Autodesk Inventor part; units mm, degrees
ref_plane "Start Plane" through (0, 0, 0) normal (0, 0, 1) x (1, 0, 0)
ref_plane "End Plane" through (0, 0, 406.9182) normal (0, 0, 1) x (1, 0, 0)
ref_plane "YZ Plane" through (0, 0, 0) normal (1, 0, 0) x (0, 1, 0)
ref_plane "Start Plane" through (0, 0, 0) normal (0, 0, 1) x (1, 0, 0)
ref_plane "End Plane" through (0, 0, 406.9182) normal (0, 0, 1) x (1, 0, 0)
sketch "Sketch" plane through (0, 0, 0) normal (0, 0, 1) x (1, 0, 0)
  line L0 (-9.525, -8.0315) -> (-9.525, 8.0315)
  line L1 (-8.0315, 9.525) -> (8.0315, 9.525)
  line L2 (9.525, 8.0315) -> (9.525, -8.0315)
  line L3 (8.0315, -9.525) -> (-8.0315, -9.525)
  arc A0 (-9.525, -8.0315) -> (-8.0315, -9.525) centre (-8.0315, -8.0315) ccw
  arc A1 (-8.0315, 9.525) -> (-9.525, 8.0315) centre (-8.0315, 8.0315) ccw
  arc A2 (9.525, 8.0315) -> (8.0315, 9.525) centre (8.0315, 8.0315) ccw
  arc A3 (8.0315, -9.525) -> (9.525, -8.0315) centre (8.0315, -8.0315) ccw
  arc A4 (-8.0315, 8.2804) -> (-8.2804, 8.0315) centre (-8.0315, 8.0315) ccw
  line L4 (-8.0315, 8.2804) -> (8.0315, 8.2804)
  arc A5 (8.2804, 8.0315) -> (8.0315, 8.2804) centre (8.0315, 8.0315) ccw
  line L5 (8.2804, 8.0315) -> (8.2804, -8.0315)
  arc A6 (8.0315, -8.2804) -> (8.2804, -8.0315) centre (8.0315, -8.0315) ccw
  line L6 (8.0315, -8.2804) -> (-8.0315, -8.2804)
  arc A7 (-8.2804, -8.0315) -> (-8.0315, -8.2804) centre (-8.0315, -8.0315) ccw
  line L7 (-8.2804, -8.0315) -> (-8.2804, 8.0315)
  line L8 (0, 13.768) -> (0, -13.768) construction
  line L9 (-13.8012, 0) -> (13.9669, 0) construction
  dimension "d10" = 19.05
  dimension "d11" = 19.05
  dimension "d12" = 1.2446
  dimension "d15" = 9.525
  dimension "d16" = 9.525
  dimension "d17" = 1.4935
extrude "Body" add sketch "Sketch" along normal up to surface (406.9182 mm away) from surface at 0
sketch "Sketch3" plane through (0, 0, 0) normal (0, 0, 1) x (1, 0, 0)
  line L0 (0, 0) -> (10, 0)
ref_plane "Work Plane3" through (0, 0, 0) normal (0, -1, 0) x (1, 0, 0)
sketch "Sketch5" plane through (9.525, -8.0315, 406.9182) normal (1, 0, 0) x (0, 0, -1)
  circle A0 centre (326.3769, 8.0315) radius 4.7702
  line L0 (0, 16.063) -> (0, 0)
  line L1 (406.9182, 0) -> (0, 0)
  line L2 (406.9182, 16.063) -> (406.9182, 0)
  line L3 (406.9182, 16.063) -> (0, 16.063)
  line L4 (406.9182, 16.063) -> (406.9182, 0)
  point P0 (406.9182, 8.0315)
  point P1 (406.9182, 8.0315)
extrude "Extrusion2" cut sketch "Sketch5" against normal through all contours A0
sketch "Sketch4" plane through (0, 0, 0) normal (0, -1, 0) x (1, 0, 0)
  line L0 (-2, 0) -> (12, 0)
  line L1 (-2, 406.9182) -> (12, 406.9182)
  dimension "d19" = 406.9182
equation "\"d10\" = G_H"
equation "\"d11\" = G_W"
equation "\"d12\" = G_T"
equation "\"d15\" = 0.5 * d10"
equation "\"d16\" = 0.5 * d11"
equation "\"d17\" = G_IR"
equation "\"d3\" = G_L"
equation "\"G_W\" = 19.05"
equation "\"G_H\" = 19.05"
equation "\"G_T\" = 1.2446"
equation "\"G_IR\" = 1.2 * G_T"
equation "\"G_L\" = d19"
equation "\"G_OFFSET_START\" = 0"
equation "\"G_OFFSET_END\" = 0"
equation "\"d14\" = G_OFFSET_END + B_L"
equation "\"B_L\" = 406.91824"
properties part number "ASTM A513 - 3/4 x 3/4 x 49/1000 - 16.02" material "Steel, Mild"
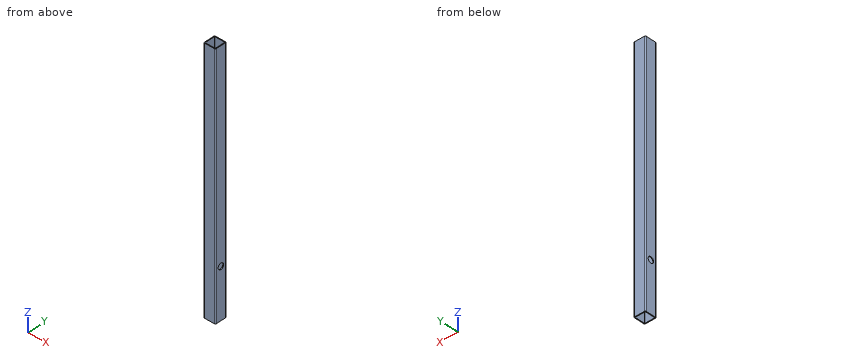
Here's how the part is built. I have some questions about the finished solid (model axes, mm). Round coordinates to 2 decimals unless told otherwise and drop trailing zeros. Loops run counter-clockwise (first coordinate to the right, second up) from the corner with the lowest first, then second, coordinate; pieces in that order, holes last.
1. If I drill on line 1 along X through (y, z) = (-7.5, 262.5) (3 decimals); line 2 along Z through (x, y) = (-8.5, -2), over which ranges is the centre line in solid material (lowest first)?
Answer list:
line 1: x = -9.525 to -8.28, 8.28 to 9.525
line 2: z = 0 to 76.21, 84.87 to 406.92
2. If we section it at A-A on x = -1.25: Write out the boundary of the cut face in (y, z) (3 decimals).
Answer list:
outline: (-9.525, 0) - (-8.28, 0) - (-8.28, 406.918) - (-9.525, 406.918) - close; (8.28, 0) - (9.525, 0) - (9.525, 406.918) - (8.28, 406.918) - close
3. For P1, Ø7.5, axis at y = 0, z = 80.54, coming from the -X side, with a flat end and sliding along its axis, tell me the tip position at first contact or that it passes through.
Answer list:
P1: passes through
4. If we section it at C-C on y = 0: Write out the boundary of the cut face in (x, z) (1 decimal), plus the area to 3 significant figures.
Answer list:
outline: (-9.5, 0) - (-8.3, 0) - (-8.3, 75.8) - (-9.5, 75.8) - close; (-9.5, 85.3) - (-8.3, 85.3) - (-8.3, 406.9) - (-9.5, 406.9) - close; (8.3, 0) - (9.5, 0) - (9.5, 75.8) - (8.3, 75.8) - close; (8.3, 85.3) - (9.5, 85.3) - (9.5, 406.9) - (8.3, 406.9) - close
area: 989 mm2
